from build123d import *

# Parameters (mm, degrees)
SKIZZE1_W                                            = 55
SKIZZE1_H                                            = 10
AUFSATZ_LINEAR_AUSTRAGEN1_DEPTH                      = 15
SCHNITT_LINEAR_AUSTRAGEN1_DEPTH                      = 15
SKIZZE3_R                                            = 1
SCHNITT_LINEAR_AUSTRAGEN2_DEPTH                      = 20
FORMSENKUNG_F_R_M4_SENKSCHRAUBE_MIT_INNE_D           = 4.5
FORMSENKUNG_F_R_M4_SENKSCHRAUBE_MIT_INNE_DEPTH       = 21.5
FORMSENKUNG_F_R_M4_SENKSCHRAUBE_MIT_INNE_CSINK_D     = 9.18
FORMSENKUNG_F_R_M4_SENKSCHRAUBE_MIT_INNE_CSINK_ANGLE = 90
FORMSENKUNG_F_R_M4_SENKSCHRAUBE_MIT_INNE_TIP         = 1.351936393


with BuildPart() as part:
    # Skizze1 → Aufsatz-Linear austragen1 (new body)
    with BuildSketch(Plane(origin=(0, 0, 0), x_dir=(1, 0, 0), z_dir=(0, 1, 0))):
        with Locations((-11.047495286, -11.601305052)):
            Rectangle(SKIZZE1_W, SKIZZE1_H)
    extrude(amount=AUFSATZ_LINEAR_AUSTRAGEN1_DEPTH)

    # Skizze2 → Schnitt-Linear austragen1 (cut)
    with BuildSketch(Plane(origin=(0, 0, 6.601305052), x_dir=(-1, 0, 0), z_dir=(0, 0, -1))):
        with BuildLine():
            Line((0.297495286, 8), (0.297495286, 0))
            Line((0.297495286, 0), (6.797495286, 0))
            Line((6.797495286, 0), (6.797495286, 8))
            ThreePointArc((6.797495286, 8), (3.547495286, 11.25), (0.297495286, 8))
        make_face()
    extrude(amount=-SCHNITT_LINEAR_AUSTRAGEN1_DEPTH, mode=Mode.SUBTRACT)

    # Skizze3 → Schnitt-Linear austragen2 (cut)
    with BuildSketch(Plane.XZ):
        with Locations(Location((-14.797495286, 11.601305052, 0), (0, 0, 270))):
            Circle(SKIZZE3_R)
        with Locations(Location((-30.547495286, 11.601305052, 0), (0, 0, 270))):
            Circle(SKIZZE3_R)
    extrude(amount=-SCHNITT_LINEAR_AUSTRAGEN2_DEPTH, mode=Mode.SUBTRACT)

    # Formsenkung für M4 Senkschraube mit Innensechskant1
    with Locations(Plane(origin=(-30.547495286, 0, 11.601305052), x_dir=(0, 0, -1), z_dir=(0, -1, 0))):
        with Locations((0, 0), (0, 15.75)):
            CounterSinkHole(FORMSENKUNG_F_R_M4_SENKSCHRAUBE_MIT_INNE_D / 2, FORMSENKUNG_F_R_M4_SENKSCHRAUBE_MIT_INNE_CSINK_D / 2, depth=FORMSENKUNG_F_R_M4_SENKSCHRAUBE_MIT_INNE_DEPTH, counter_sink_angle=FORMSENKUNG_F_R_M4_SENKSCHRAUBE_MIT_INNE_CSINK_ANGLE)
            with Locations((0, 0, -(FORMSENKUNG_F_R_M4_SENKSCHRAUBE_MIT_INNE_DEPTH + FORMSENKUNG_F_R_M4_SENKSCHRAUBE_MIT_INNE_TIP / 2))):  # 118° drill point
                Cone(0, FORMSENKUNG_F_R_M4_SENKSCHRAUBE_MIT_INNE_D / 2, FORMSENKUNG_F_R_M4_SENKSCHRAUBE_MIT_INNE_TIP, mode=Mode.SUBTRACT)


solid = part.part
The listing builds one solid part. Answer for the finished solid, in the listing's coordinates (mm). A direction names the side the tool comes from. Coordinates: 2 decimals unless noted, no trailing zeros. Write each loop counter-clockwise with the first axis right and the second up, starting at its lowest first coordinate (ties: lowest second). Pieces come first, ordered by that corner, then holes. Notation, with made-up numbers: (60.25, 64) - (78.25, 64) arc R18 cw to (78.25, 77) - close; hole circle Ø9 at (84.5, 24). An arc over 180 degrees is marked (long way). Return JSON: item names as keys, results as strings.
1. This flat-tipped pin is pushed along its axis until it touches: pin 1 Ø1 at (x, z) = (-1.5, 15) entering from -Y. Where does it stop, or does it pass through?
Final values:
{"pin 1": "y = 10.02"}
2. Which of the six approach directions +Z, -Z, +X, -X, +Y, -Y give full straight-line access (tool end or side, diameter ignored) to faces 4 (the face through (-23, 0, 12)), 5 (the face through (-0.297, 4, 12))?
Final values:
{"face 4": "+Z, -Z, +X, -X, -Y", "face 5": "+Z, -Z, -Y"}
3. The part is cut by section B-B on y = 6. Determine the outline of the cut face in (x, z).
Final values:
{"outline": "(-38.55, 6.6) - (-6.8, 6.6) - (-6.8, 16.6) - (-38.55, 16.6) - close; (-0.3, 6.6) - (16.45, 6.6) - (16.45, 16.6) - (-0.3, 16.6) - close; hole circle Ø4.5 at (-30.55, 11.6); hole circle Ø4.5 at (-14.8, 11.6)"}
4. The part is cut by section C-C on z = 12.75. Count the separate pieces of the cut face and the enclosed holes in it, then the cut area to 3 significant figures.
Final values:
{"separate pieces": "3", "enclosed holes": "0", "area": "628 mm^2"}
5. For a pull along Z with two mould halves and no side action, classify faces 1 (the face through (8, 0, 12)), 2 (the face through (-16.24, 2.23, 9.73)), 3 (the face through (-11, 7, 16.601)) as +Z half, -Z half, draft (parallel to the pull), parting line (faces both ways), or undercut.
Final values:
{"face 1": "draft", "face 2": "undercut", "face 3": "+Z half"}
6. The part is cut by section D-D on y = 13.5. Determine the outline of the cut face in (x, z).
Final values:
{"outline": "(-38.55, 6.6) - (16.45, 6.6) - (16.45, 16.6) - (-38.55, 16.6) - close; hole circle Ø4.5 at (-30.55, 11.6); hole circle Ø4.5 at (-14.8, 11.6)"}
7. The part is cut by section A-A on y = 1.75. Determine the outline of the cut face in (x, z).
Final values:
{"outline": "(-38.55, 6.6) - (-6.8, 6.6) - (-6.8, 16.6) - (-38.55, 16.6) - close; (-0.3, 6.6) - (16.45, 6.6) - (16.45, 16.6) - (-0.3, 16.6) - close; hole circle Ø5.68 at (-30.55, 11.6); hole circle Ø5.68 at (-14.8, 11.6)"}
8. Consider line 1 along X through (y, z) = (7.25, 9); line 2 along Z through (x, y) = (-15, 5.5); line 3 along X through (y, z) = (12.5, 10.75). Determine where each line is inside the solid, lowest interval first.
Final values:
{"line 1": "-38.55 to -6.8, -0.3 to 16.45", "line 2": "6.6 to 9.36, 13.84 to 16.6", "line 3": "-38.55 to -32.63, -28.46 to -16.88, -12.71 to 16.45"}
